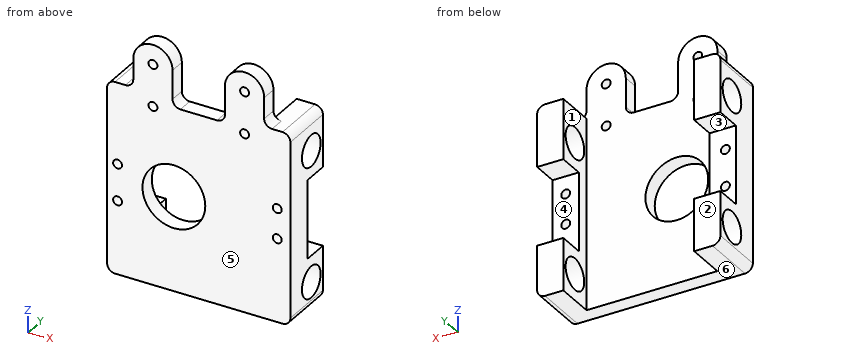
```python
from build123d import *

# Parameters (mm, degrees)
ESQUISSE1_R             = 12
BOSS_EXTRU_1_DEPTH      = 6
ESQUISSE3_W             = 10
ESQUISSE3_H             = 73
BOSS_EXTRU_2_DEPTH      = 15
ESQUISSE4_R             = 6
ESQUISSE4_W             = 30
ESQUISSE4_H             = 10
ENL_V_MAT_EXTRU_1_DEPTH = 71
D_GAGEMENT_M32_D        = 3.4
D_GAGEMENT_M32_DEPTH    = 11
CONG_2_R                = 3


with BuildPart() as part:
    # Esquisse1 → Boss.-Extru.1 (new body)
    with BuildSketch(Plane(origin=(0, 0, 0), x_dir=(1, 0, 0), z_dir=(0, 1, 0))):
        with BuildLine():
            Line((0, 0), (70, 0))
            Line((70, 0), (70, -73))
            Line((70, -73), (60, -73))
            Line((60, -73), (60, -84))
            ThreePointArc((60, -84), (52.5, -91.5), (45, -84))
            Line((45, -84), (45, -70))
            Line((45, -70), (25, -70))
            Line((25, -70), (25, -84))
            ThreePointArc((25, -84), (17.5, -91.5), (10, -84))
            Line((10, -84), (10, -73))
            Line((10, -73), (0, -73))
            Line((0, -73), (0, 0))
        make_face()
        with Locations((25.5, -36)):
            Circle(ESQUISSE1_R, mode=Mode.SUBTRACT)
    extrude(amount=BOSS_EXTRU_1_DEPTH)

    # Esquisse3 → Boss.-Extru.2 (add)
    with BuildSketch(Plane(origin=(0, 6, 0), x_dir=(1, 0, 0), z_dir=(0, 1, 0))):
        with Locations((5, -36.5)):
            Rectangle(ESQUISSE3_W, ESQUISSE3_H)
        with Locations((65, -36.5)):
            Rectangle(ESQUISSE3_W, ESQUISSE3_H)
    extrude(amount=BOSS_EXTRU_2_DEPTH)

    # Esquisse4 → Enlèv. mat.-Extru.1 (cut, through all)
    with BuildSketch(Plane(origin=(0, 0, 0), x_dir=(0, 0, -1), z_dir=(1, 0, 0))):
        with Locations((-60, 13.5)):
            Circle(ESQUISSE4_R)
        with Locations((-10, 13.5)):
            Circle(ESQUISSE4_R)
        with Locations((-35, 16)):
            Rectangle(ESQUISSE4_W, ESQUISSE4_H)
    extrude(amount=ENL_V_MAT_EXTRU_1_DEPTH, mode=Mode.SUBTRACT)

    # Dégagement M32
    with Locations(Plane(origin=(0, 11, 0), x_dir=(1, 0, 0), z_dir=(0, 1, 0))):
        with Locations((4, -28), (4, -42), (17.5, -84), (52.5, -84), (17.5, -68), (52.5, -68), (65, -31.75), (65, -43.25)):
            Hole(D_GAGEMENT_M32_D / 2, depth=D_GAGEMENT_M32_DEPTH)

    # Congé2
    cong_2_edges = [part.edges().sort_by_distance(p)[0] for p in [
        (0, 10.5, 0),
        (70, 10.5, 0),
        (70, 10.5, 73),
        (60, 3, 73),
        (45, 3, 70),
        (25, 3, 70),
        (10, 3, 73),
        (0, 10.5, 73),
    ]]
    fillet(cong_2_edges, radius=CONG_2_R)


solid = part.part
```
Read the model definition and answer for the solid it produces. Units are mm, in the model's axes. Face numbers are marked on the shaded views. A direction names the side the tool comes from. Give positions to 0.01 mm unless a question says otherwise; leave off trailing zeros. Write each loop counter-clockwise with the first axis right and the second up, starting at its lowest first coordinate (ties: lowest second). Pieces come first, ordered by that corner, then holes. Notation, with made-up numbers: M 86,33.5 L 130,33.5 A19 cw 130,64.5 Z; hole C 45.5,83.25 d9. An arc over 180 degrees is marked long. Put each result on its own line as item: value. Start each with the question number.
1. Which of the six approach directions +Z, -Z, +X, -X, +Y, -Y give full straight-line access (tool end or side, diameter ignored) to the marked faces 1, 2 and 3?
2. The part is cut by section A-A, the plane z = 68. Give the vertices of the cut face in (x, y).
3. For a pull along Z with two mould halves and no side action, classify the marked faces 4, 5 and 6 as released by +Z, released by -Z, zero draft, split by the parting line, or undercut.
4. The part is cut by section C-C, the plane y = 2. Give the number of separate pieces and of enclosed holes in the cut face, and give its area (3 significant figures).
5. The part is cut by section B-B, the plane x = 52.5. Give the vertices of the cut face in (y, z).
6. Each of these flat-tipped pins is pushed along its axis until it touches: pin 1 Ø5.5 at (x, z) = (65, 31.75) entering from -Y; pin 2 Ø5.5 at (x, z) = (17.5, 68) entering from +Y; pin 3 Ø7.5 at (x, y) = (7, 10.5) entering from +Z; pin 4 Ø5 at (y, z) = (3.5, 80.5) entering from +X. Where does it stop, or does it pass through?
7. The part is cut by section D-D, the plane x = 4. Give the vertices of the cut face in (y, z).
8. Consider line 1 along Z through (x, y) = (4, 3.25); line 2 along X through (y, z) = (4.6, 84); line 3 along Y through (x, z) = (5, 60). Determine where each line is inside the solid, lowest interval first.
Final values:
1. face 1: +Z, -Z, +Y
1. face 2: +Z, -Z, +X, -X, +Y
1. face 3: +X, -X, +Y
2. outline: M 0,0 L 15.8,0 L 15.8,6 L 10,6 L 10,21 L 0,21 Z; M 19.2,0 L 50.8,0 L 50.8,6 L 19.2,6 Z; M 54.2,0 L 70,0 L 70,21 L 60,21 L 60,6 L 54.2,6 Z
3. face 4: undercut
3. face 5: zero draft
3. face 6: released by -Z
4. separate pieces: 1
4. enclosed holes: 9
4. area: 5,030 mm²
5. outline: M 0,0 L 6,0 L 6,66.3 L 0,66.3 Z; M 0,69.7 L 6,69.7 L 6,82.3 L 0,82.3 Z; M 0,85.7 L 6,85.7 L 6,91.5 L 0,91.5 Z
6. pin 1: stops at y = 0
6. pin 2: stops at y = 6
6. pin 3: stops at z = 73
6. pin 4: stops at x = 60
7. outline: M 0,0 L 21,0 L 21,20 L 11,20 L 11,26.3 L 0,26.3 Z; M 0,29.7 L 11,29.7 L 11,40.3 L 0,40.3 Z; M 0,43.7 L 11,43.7 L 11,50 L 21,50 L 21,73 L 0,73 Z; hole C 13.5,10 d12; hole C 13.5,60 d12
8. line 1: z = 0 to 26.3, 29.7 to 40.3, 43.7 to 73
8. line 2: x = 10 to 15.8, 19.2 to 25, 45 to 50.8, 54.2 to 60
8. line 3: y = 0 to 7.5, 19.5 to 21
